Autodesk Inventor part; units mm, degrees
ref_plane "YZ Plane" through (0, 0, 0) normal (1, 0, 0) x (0, 1, 0)
ref_plane "XZ Plane" through (0, 0, 0) normal (0, 1, 0) x (-1, 0, 0)
ref_plane "XY Plane" through (0, 0, 0) normal (0, 0, 1) x (1, 0, 0)
sketch "Skizze1" plane through (0, 0, 0) normal (1, 0, 0) x (0, 1, 0)
  line L0 (4, 0) -> (4, 3)
  arc A0 (4, 3) -> (3, 4) centre (3, 3) ccw
  line L1 (3, 4) -> (0, 4)
  line L2 (0, 4) -> (0, 5)
  line L3 (0, 5) -> (-3, 5)
  line L4 (-3, 5) -> (-3, 2)
  line L5 (0, 0) -> (4, 0)
  line L6 (-3, 2) -> (-3, 0)
  line L7 (-3, 0) -> (0, 0)
  point P0 (0, 2)
  dimension "d0" = 2
  dimension "d1" = 4
  dimension "d2" = 3
  dimension "d3" = 5
  dimension "d4" = 3
  dimension "d5" = 1
  dimension "d6" = 1
revolve "Umdrehung1" add sketch "Skizze1" angle 360 about axis through (0, 0, 0) along (0, 1, 0)
sketch "Skizze2" plane through (0, 4, 0) normal (0, 1, 0) x (1, 0, 0)
  line L0 (-1.7168, -1.418) -> (-1.7168, 1.5147) construction
  line L1 (-1.7168, 1.5147) -> (1.7832, 1.5147) construction
  line L2 (1.7832, 1.5147) -> (1.7832, -1.418) construction
  line L3 (1.7832, -1.418) -> (-1.7168, -1.418) construction
  line L4 (1.7832, 1.3559) -> (1.7832, 0.8227)
  line L5 (1.7832, 0.8227) -> (0.3877, -0.0282)
  line L6 (0.3877, -0.0282) -> (1.7832, -0.8961)
  line L7 (1.7832, -0.8961) -> (1.7832, -1.3981)
  line L8 (1.7832, -1.3981) -> (0.0304, -0.2835)
  line L9 (0.0304, -0.2835) -> (-1.7168, -1.3641)
  line L10 (-1.7168, -1.3641) -> (-1.7168, -0.8309)
  line L11 (-1.7168, -0.8309) -> (-0.3469, 0.003)
  line L12 (-0.3469, 0.003) -> (-1.7168, 0.8539)
  line L13 (-1.7168, 0.8539) -> (-1.7168, 1.3559)
  line L14 (-1.7168, 1.3559) -> (0.0077, 0.2611)
  line L15 (0.0077, 0.2611) -> (1.7832, 1.3559)
  point P0 (0, 0)
extrude "Extrusion1" cut sketch "Skizze2" against normal blind 0.5
sketch "Skizze4" plane through (0, -3, 0) normal (0, -1, 0) x (1, 0, 0)
  line L0 (4.8726, 0.75) -> (6.8726, 0.75)
  line L1 (6.8726, 0.75) -> (6.8726, -0.75)
  line L2 (6.8726, -0.75) -> (4.8726, -0.75)
  line L3 (4.8726, -0.75) -> (4.8726, 0.75)
  point P0 (0, 0)
  dimension "d15" = 1.5
  dimension "d16" = 2
  dimension "d17" = 0.75
extrude "Extrusion3" add sketch "Skizze4" against normal blind 3
properties part number "ButtonX_neu"
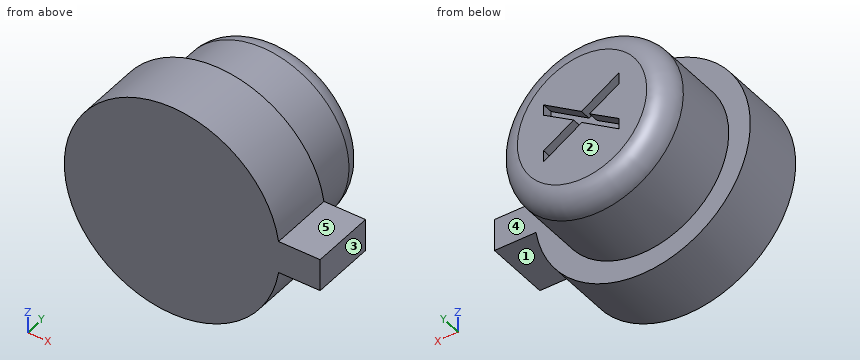
CAD build for the part. Positions are in the model's coordinates, mm. Face numbers are marked on the shaded views. A direction names the side the tool comes from. Round coordinates to 2 decimals unless told otherwise and drop trailing zeros. Loops run counter-clockwise (first coordinate to the right, second up) from the corner with the lowest first, then second, coordinate; pieces in that order, holes last. Notation, with made-up numbers: (32, 69.25) - (72, 69.25) arc R15 cw to (72, 77.25) - close; hole circle Ø11 at (28, -11.75). An arc over 180 degrees is marked (long way). Return JSON: item names as keys, results as strings. Group by question number.
Q1. Flat gauge pins, fed straight in: pin 1 Ø1.5 at (x, y) = (6, -2) entering from -Z; pin 2 Ø2 at (x, y) = (3.5, -1) entering from +Z; pin 3 Ø0.6 at (x, y) = (5.5, -1) entering from +Z; pin 4 Ø1.4 at (x, z) = (0.5, 0.5) entering from +Y. Where does each tip first touch, or does it go through?
Q2. Drill centre lines: line 1 along Y through (x, z) = (4.5, -1.5); line 2 along Y through (x, z) = (-2.5, -1.75); line 3 along X through (y, z) = (-2.5, 4). Where is each one in solid material? Low to high. Write a range as [from, to].
Q3. Band-saw the part on C-C on y = -0.75. Give the cut face in (x, z).
Q4. Band-saw the part on A-A on y = 3.75. Give the cut face in (x, z), plus the area to 3 significant figures.
Q5. Tool access for the marked faces 1, 2, 3, 4 and 5: list every direction of +Z, -Z, +X, -X, +Y, -Y with a clear straight run to the whole face (end or side of a thin tool).
Q6. Band-saw the part on B-B on x = 5.75. Give the cut face in (y, z), plus the area to 3 significant figures.
Q7. Band-saw the part on D-D on y = 2.5. Give the cut face in (x, z).
Solutions:
{
 "1": {"pin 1": "stops at z = -0.75", "pin 2": "stops at z = 4.33", "pin 3": "stops at z = 0.75", "pin 4": "stops at y = 4"},
 "2": {"line 1": "y = [-3, 0]", "line 2": "y = [-3, 4]", "line 3": "x = [-3, 3]"},
 "3": {"outline": "(4.94, -0.75) - (6.87, -0.75) - (6.87, 0.75) - (4.94, 0.75) arc R5 ccw (long way) to start"},
 "4": {"outline": "circle Ø7.32 at (0, 0); hole (-1.72, -1.36) - (0.01, -0.26) - (1.78, -1.36) - (1.78, -0.82) - (0.39, 0.03) - (1.78, 0.9) - (1.78, 1.4) - (0.03, 0.28) - (-1.72, 1.36) - (-1.72, 0.83) - (-0.35, 0) - (-1.72, -0.85) - close", "area": "38.7 mm^2"},
 "5": {"face 1": "-Z, +X, +Y, -Y", "face 2": "+Z, -Z, +X, -X, +Y", "face 3": "+Z, -Z, +X, +Y, -Y", "face 4": "+Y", "face 5": "+Z, +X, +Y, -Y"},
 "6": {"outline": "(-3, -0.75) - (0, -0.75) - (0, 0.75) - (-3, 0.75) - close", "area": "4.50 mm^2"},
 "7": {"outline": "circle Ø8 at (0, 0)"}
}
